```python
from build123d import *

# Parameters (mm, degrees)
SKETCH2_W           = 226.314
SKETCH2_H           = 215.9
BOSS_EXTRUDE1_DEPTH = 12.7
SKETCH3_W           = 12.7
SKETCH3_H           = 25.4
BOSS_EXTRUDE2_DEPTH = 12.7
SKETCH4_R           = 6.35
SKETCH4_R_2         = 3.81
CUT_EXTRUDE1_DEPTH  = 12.7
SKETCH5_W           = 226.314
SKETCH5_H           = 12.7
BOSS_EXTRUDE3_DEPTH = 12.7


with BuildPart() as part:
    # Sketch2 → Boss-Extrude1 (new body)
    with BuildSketch(Plane.XY):
        with Locations((-9.264561791, -20.772712934)):
            Rectangle(SKETCH2_W, SKETCH2_H)
    extrude(amount=BOSS_EXTRUDE1_DEPTH)

    # Sketch3 → Boss-Extrude2 (add)
    with BuildSketch(Plane(origin=(103.892438209, 0, 0), x_dir=(0, 0, -1), z_dir=(1, 0, 0))):
        with Locations((-6.35, -14.422712934)):
            Rectangle(SKETCH3_W, SKETCH3_H)
    extrude(amount=BOSS_EXTRUDE2_DEPTH)

    # Sketch4 → Cut-Extrude1 (cut)
    with BuildSketch(Plane(origin=(0, 0, 0), x_dir=(-1, 0, 0), z_dir=(0, 0, -1))):
        with Locations((109.721561791, -14.422712934)):
            Circle(SKETCH4_R)
        with Locations((-110.242438209, -8.072712934)):
            Circle(SKETCH4_R_2)
        with Locations((-110.242438209, -20.772712934)):
            Circle(SKETCH4_R_2)
    extrude(amount=-CUT_EXTRUDE1_DEPTH, mode=Mode.SUBTRACT)

    # Sketch5 → Boss-Extrude3 (add)
    with BuildSketch(Plane(origin=(0, 87.177287066, 0), x_dir=(1, 0, 0), z_dir=(0, 1, 0))):
        with Locations((-9.264561791, -6.35)):
            Rectangle(SKETCH5_W, SKETCH5_H)
    extrude(amount=BOSS_EXTRUDE3_DEPTH)


solid = part.part
```
Verification items for the finished model (mm, model axes). A direction names the side the tool comes from. Round coordinates to 2 decimals unless told otherwise and drop trailing zeros. Order: outer loops, then holes, each group sorted by start corner. A loop starts at its lowest first (then second) coordinate and runs counter-clockwise, first axis right, second up.
1) Depth check by flat-ended pin: pin 1 (6.5 mm diameter, centred on y = 28.5, z = 4.5, fed in from +X); pin 2 (11.5 mm diameter, centred on x = -109.72, y = -14.42, fed in from -Z); pin 3 (4 mm diameter, centred on x = 107.5, z = 3.5, fed in from +Y). Enter the tip coordinate at first touch or a pass-through.
Geometry says:
pin 1: stops at x = 103.89
pin 2: passes through
pin 3: stops at y = -1.72
2) Draft check along X on faces 1 (the flat face through (-11, -128.723, 6)), 2 (the flat face through (-122.422, -16, 6)), 3 (the cylindrical face through (-103.378, -14.144, 6.261)). Enter one of: +X half, -X half, draft (parallel to the pull), parting line (faces both ways), or undercut.
Geometry says:
face 1: draft
face 2: -X half
face 3: undercut
3) Cross-section at B-B, the plane y = -100. Record the cut outline in (x, z).
Geometry says:
outline: (-122.42, 0) - (103.89, 0) - (103.89, 12.7) - (-122.42, 12.7) - close
4) Material ranges on line 1 (X direction, y = 75, z = 8); line 2 (Y direction, x = -106, z = 5.5); line 3 (X direction, y = -16, z = 7.5), recorded low to high.
Geometry says:
line 1: x = -122.42 to 103.89
line 2: y = -128.72 to -19.57, -9.28 to 99.88
line 3: x = -122.42 to -115.87, -103.57 to 116.59
5) Tool access check on faces 4 (the cylindrical face through (106.608, -6.928, 6.261)), 5 (the flat face through (110, -1.723, 6)), 6 (the flat face through (103.892, -79, 6)). Record the directions out of +Z, -Z, +X, -X, +Y, -Y that give a thin tool (end or side, any length) a straight path to the whole face; none if there is none.
Geometry says:
face 4: +Z, -Z
face 5: +Z, -Z, +X, +Y
face 6: +Z, -Z, +X, -Y
6) Cross-section at A-A, the plane z = 10.5. Record the cut outline in (x, y), plus the area to 3 significant figures.
Geometry says:
outline: (-122.42, -128.72) - (103.89, -128.72) - (103.89, -27.12) - (116.59, -27.12) - (116.59, -1.72) - (103.89, -1.72) - (103.89, 99.88) - (-122.42, 99.88) - close; hole circle Ø12.7 at (-109.72, -14.42); hole circle Ø7.62 at (110.24, -20.77); hole circle Ø7.62 at (110.24, -8.07)
area: 51,800 mm2
